Autodesk Inventor part; units mm, degrees
ref_plane "YZ Plane" through (0, 0, 0) normal (1, 0, 0) x (0, 1, 0)
ref_plane "XZ Plane" through (0, 0, 0) normal (0, 1, 0) x (-1, 0, 0)
ref_plane "XY Plane" through (0, 0, 0) normal (0, 0, 1) x (1, 0, 0)
sketch "Sketch1" plane through (0, 0, 0) normal (0, 1, 0) x (-1, 0, 0)
  line L0 (-8.185, 14.605) -> (8.185, 14.605)
  line L1 (8.185, 14.605) -> (8.185, -14.605)
  line L2 (8.185, -14.605) -> (-8.185, -14.605)
  line L3 (-8.185, -14.605) -> (-8.185, 14.605)
  line L4 (-8.185, 14.605) -> (8.185, -14.605) construction
  line L5 (8.185, 14.605) -> (-8.185, -14.605) construction
  point P0 (0, 0)
  dimension "d0" = 16.37
  dimension "d1" = 29.21
extrude "Extrusion1" add sketch "Sketch1" along normal blind 12.4
sketch "Sketch2" plane through (-8.185, 0, 14.605) normal (0, 0, 1) x (1, 0, 0)
  line L0 (16.37, 0) -> (0, 0)
  line L1 (16.37, 0) -> (16.37, 12.4)
  line L2 (0, 12.4) -> (16.37, 12.4)
  line L3 (0, 0) -> (0, 12.4)
  line L4 (0, 12.4) -> (16.37, 12.4)
  line L5 (16.37, 12.4) -> (0, 0) construction
  line L6 (0, 12.4) -> (16.37, 0) construction
  line L7 (1.785, 1.55) -> (14.585, 1.55)
  line L8 (14.585, 1.55) -> (14.585, 10.85)
  line L9 (14.585, 10.85) -> (1.785, 10.85)
  line L10 (1.785, 10.85) -> (1.785, 1.55)
  line L11 (1.785, 1.55) -> (14.585, 10.85) construction
  line L12 (14.585, 1.55) -> (1.785, 10.85) construction
  point P0 (8.185, 0)
  point P1 (8.185, 6.2)
  dimension "d4" = 12.8
  dimension "d5" = 9.3
extrude "Extrusion2" cut sketch "Sketch2" against normal blind 11.41
sketch "Sketch3" plane through (8.185, 0, -14.605) normal (0, 0, -1) x (-1, 0, 0)
  line L0 (16.37, 0) -> (0, 0)
  line L1 (16.37, 0) -> (16.37, 12.4)
  line L2 (0, 12.4) -> (16.37, 12.4)
  line L3 (0, 0) -> (0, 12.4)
  line L4 (1.785, 10.85) -> (14.585, 10.85)
  line L5 (1.785, 1.55) -> (1.785, 10.85)
  line L6 (14.585, 1.55) -> (1.785, 1.55)
  line L7 (14.585, 10.85) -> (14.585, 1.55)
  line L8 (15.335, 11.6) -> (1.035, 11.6)
  line L9 (1.035, 11.6) -> (1.035, 0.8)
  line L10 (1.035, 0.8) -> (15.335, 0.8)
  line L11 (15.335, 0.8) -> (15.335, 11.6)
  point P0 (8.185, 0)
  dimension "d8" = 10.8
extrude "Extrusion3" cut sketch "Sketch3" against normal blind 16.46 contours L0 L3 L2 L1
sketch "Sketch4" plane through (7.15, 0.8, -14.605) normal (0, 0, -1) x (-1, 0, 0)
  line L0 (0.75, 10.05) -> (13.55, 10.05)
  line L1 (13.55, 10.05) -> (13.55, 0.75)
  line L2 (13.55, 0.75) -> (0.75, 0.75)
  line L3 (0.75, 0.75) -> (0.75, 10.05)
  line L4 (0, 10.8) -> (0, 0)
  line L5 (0, 0) -> (14.3, 0)
  line L6 (14.3, 0) -> (14.3, 10.8)
  line L7 (14.3, 10.8) -> (0, 10.8)
  point P0 (7.15, -0.8)
extrude "Extrusion4" cut sketch "Sketch4" against normal blind 12.75
sketch "Sketch5" plane through (6.4, 1.55, -14.605) normal (1, 0, 0) x (0, 0, -1)
  line L0 (-29.21, 0) -> (-29.21, 9.3)
  line L1 (-29.21, 0) -> (-17.8, 0)
  line L2 (-17.8, 0) -> (-17.8, 9.3)
  line L3 (-29.21, 9.3) -> (-17.8, 9.3)
  line L4 (0, 9.3) -> (0, 0)
  line L5 (0, 9.3) -> (-12.75, 9.3)
  line L6 (-12.75, 9.3) -> (-12.75, 0)
  line L7 (0, 0) -> (-12.75, 0)
  circle A0 centre (-29.21, 9.3) radius 3
  line L8 (0, 0) -> (0, 9.3)
  circle A1 centre (0, 9.3) radius 3
  point P0 (-14.605, -1.55)
  dimension "d13" = 6
  dimension "d14" = 6
extrude "Extrusion5" cut sketch "Sketch5" against normal through all contours A0 L3 L0 | L0 L3 A0 | L5 A1 L4 | L4 A1 L5
sketch "Sketch6" plane through (6.4, 1.55, -14.605) normal (0, 0, -1) x (-1, 0, 0)
  line L0 (0, 9.3) -> (12.8, 9.3)
  line L1 (0, 6.3) -> (0, 9.3)
  line L2 (0, 6.3) -> (0, 0)
  line L3 (12.8, 0) -> (12.8, 6.3)
  line L4 (12.8, 9.3) -> (12.8, 6.3)
  line L5 (0, 0) -> (12.8, 0)
  line L6 (11.8, 8.3) -> (1, 8.3)
  line L7 (1, 8.3) -> (1, 6.3)
  line L8 (1, 6.3) -> (1, 1)
  line L9 (1, 1) -> (11.8, 1)
  line L10 (11.8, 1) -> (11.8, 6.3)
  line L11 (11.8, 6.3) -> (11.8, 8.3)
  line L12 (1, 8.3) -> (11.8, 1) construction
  line L13 (1, 1) -> (11.8, 8.3) construction
  line L14 (5.9, 1) -> (6.9, 1)
  line L15 (6.9, 1) -> (6.9, 8.3)
  line L16 (6.9, 8.3) -> (5.9, 8.3)
  line L17 (5.9, 8.3) -> (5.9, 1)
  line L18 (5.9, 1) -> (6.9, 8.3) construction
  line L19 (6.9, 1) -> (5.9, 8.3) construction
  point P0 (6.4, -1.55)
  point P1 (6.4, 4.65)
  dimension "d17" = 1
  dimension "d18" = 1
extrude "Extrusion6" cut sketch "Sketch6" against normal through all contours L11 L10 L9 L15 L6 | L17 L9 L8 L7 L6
fillet "Fillet1" radius 1 12 edges at (7.15, 11.6, 0) (6.4, 10.85, -6.73) (-7.15, 11.6, 0) (-6.4, 10.85, -6.73) (6.4, 10.85, 7.4) (6.4, 1.55, 8.9) (6.4, 1.55, -8.23) (-6.4, 1.55, -8.23) (-7.15, 0.8, 0) (7.15, 0.8, 0) (-6.4, 1.55, 8.9) (-6.4, 10.85, 7.4)
properties part number "lcLcCoupler" material "Stainless Steel"
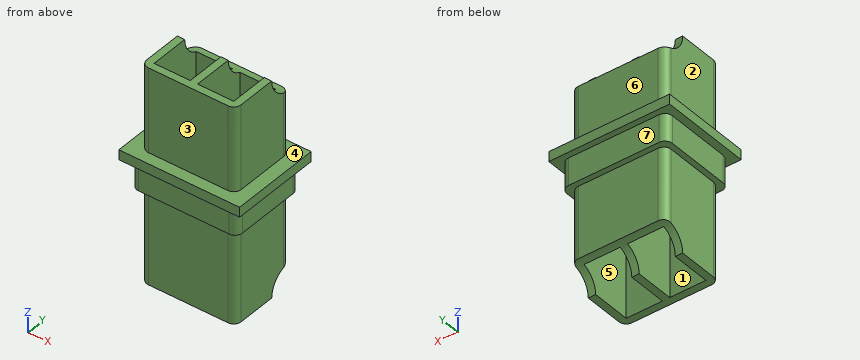
Can you work these out from the model? Positions are in its coordinate system, mm. Face numbers are marked on the shaded views. A direction names the side the tool comes from. Give positions to 0.01 mm unless a question says otherwise; leave off trailing zeros. Loops run counter-clockwise (first coordinate to the right, second up) from the corner with the lowest first, then second, coordinate; pieces in that order, holes last. Notation, with made-up numbers: M 52,-28 L 100,-28 A16 ccw 100,-1 Z; hole C 82,-9 d8. An arc over 180 degrees is marked long. One line per item, written item: value. Start each with the question number.
1) If we section it at D-D, the plane z = 10.5: Write out the boundary of the cut face in (x, y).
2) If we section it at A-A, the plane y = 3: Write out the boundary of the cut face in (x, z) (3 decimals).
3) If we section it at B-B, the plane x = 2: Write out the boundary of the cut face in (y, z) (3 decimals).
4) On a 3-axis mill with a long thin cutter (end or side, diameter ignored), from which of +Z, -Z, +X, -X, +Y, -Y can I reach the whole of each face in a straight line? I mean the marked faces 4, 5, 6 and 7. Say none if no direction works.
5) Thinking about a two-plate mould opening in Y: for the marked faces 1, 2 and 3, which applies, +Y half, -Y half, draft (parallel to the pull), parting line (faces both ways), or undercut?
6) I'm going to push flat-ended pins straight in: pin 1 (2 mm diameter, centred on y = 6.5, z = -2.5, fed in from -X); pin 2 (3 mm diameter, centred on x = -2.5, z = -9, fed in from +Y); pin 3 (5.5 mm diameter, centred on x = -3.5, z = -1.5, fed in from +Y); pin 4 (3 mm diameter, centred on x = 2.5, y = 5, fed in from -Z). Where does each tip first touch, or does it pass through?
7) If I drill on line 1 (X direction, y = 9.75, z = 3) (3 decimals); line 2 (X direction, y = 3.25, z = 6); line 3 (Y direction, x = -1, z = 8.5), over which ranges is the centre line in solid material (lowest first)? Write a range as [from, to].
8) If we section it at C-C, the plane z = 2.25: Write out the boundary of the cut face in (x, y) (3 decimals), and give its area (3 significant figures).
Completed:
1. outline: M -6.4,2.55 A1 ccw -5.4,1.55 L 5.4,1.55 A1 ccw 6.4,2.55 L 6.4,9.85 A1 ccw 5.4,10.85 L -5.4,10.85 A1 ccw -6.4,9.85 Z; hole M -5.4,2.55 L -0.5,2.55 L -0.5,9.85 L -5.4,9.85 Z; hole M 0.5,2.55 L 5.4,2.55 L 5.4,9.85 L 0.5,9.85 Z
2. outline: M -8.185,1.855 L -7.15,1.855 L -7.15,-1.855 L -6.4,-1.855 L -6.4,-14.605 L -5.4,-14.605 L -5.4,14.605 L -6.4,14.605 L -6.4,3.195 L -8.185,3.195 Z; M -0.5,-14.605 L 0.5,-14.605 L 0.5,14.605 L -0.5,14.605 Z; M 5.4,-14.605 L 6.4,-14.605 L 6.4,-1.855 L 7.15,-1.855 L 7.15,1.855 L 8.185,1.855 L 8.185,3.195 L 6.4,3.195 L 6.4,14.605 L 5.4,14.605 Z
3. outline: M 0,1.855 L 0.8,1.855 L 0.8,-1.855 L 1.55,-1.855 L 1.55,-14.605 L 2.55,-14.605 L 2.55,14.605 L 1.55,14.605 L 1.55,3.195 L 0,3.195 Z; M 9.85,-11.777 A3 cw 10.85,-11.605 L 10.85,-1.855 L 11.6,-1.855 L 11.6,1.855 L 12.4,1.855 L 12.4,3.195 L 10.85,3.195 L 10.85,11.605 A3 cw 9.85,11.777 Z
4. face 4: +Z
4. face 5: +Z, -Z
4. face 6: +Z, +X, -X, +Y
4. face 7: -Z, +X, -X, +Y
5. face 1: undercut
5. face 2: draft
5. face 3: -Y half
6. pin 1: stops at x = -7.15
6. pin 2: stops at y = 10.85
6. pin 3: stops at y = 11.6
6. pin 4: passes through
7. line 1: x = [-8.185, -5.4], [-0.5, 0.5], [5.4, 8.185]
7. line 2: x = [-6.4, -5.4], [-0.5, 0.5], [5.4, 6.4]
7. line 3: y = [1.55, 2.55], [9.85, 10.85]
8. outline: M -8.185,0 L 8.185,0 L 8.185,12.4 L -8.185,12.4 Z; hole M -5.4,2.55 L -0.5,2.55 L -0.5,9.85 L -5.4,9.85 Z; hole M 0.5,2.55 L 5.4,2.55 L 5.4,9.85 L 0.5,9.85 Z
8. area: 131 mm^2
